CAD build for the part. Positions are in the model's coordinates, mm. Round coordinates to 2 decimals unless told otherwise and drop trailing zeros. Loops run counter-clockwise (first coordinate to the right, second up) from the corner with the lowest first, then second, coordinate; pieces in that order, holes last.
from build123d import *

# Parameters (mm, degrees)
CYLINDER080_R     = 1.5
CYLINDER080_DEPTH = 10
CYLINDER075_R     = 2.579687
CYLINDER075_DEPTH = 56.5
CYLINDER076_R     = 2.579687
CYLINDER076_DEPTH = 55.5
BOX006_W          = 6.35
BOX006_H          = 15
BOX006_DEPTH      = 10
FILLET005_R       = 1
BOX005_W          = 6.35
BOX005_H          = 15
BOX005_DEPTH      = 10
FILLET004_R       = 1
BOX004_W          = 68
BOX004_H          = 15
BOX004_DEPTH      = 1.01
FILLET003_R       = 2


with BuildPart() as shieldcrosshole004:
    # Cylinder080 → Cylinder080 (new body)
    with BuildSketch(Plane(origin=(105, 116, 34), x_dir=(1, 0, 0), z_dir=(0, 0, 1))):
        Circle(CYLINDER080_R)
    extrude(amount=CYLINDER080_DEPTH)


with BuildPart() as threaded027:
    # Cylinder075 → Cylinder075 (new body)
    with BuildSketch(Plane(origin=(73.25, 179.75, 4), x_dir=(1, 0, 0), z_dir=(0, 0, 1))):
        Circle(CYLINDER075_R)
    extrude(amount=CYLINDER075_DEPTH)


with BuildPart() as threaded028:
    # Cylinder076 → Cylinder076 (new body)
    with BuildSketch(Plane(origin=(136.75, 179.75, 4), x_dir=(1, 0, 0), z_dir=(0, 0, 1))):
        Circle(CYLINDER076_R)
    extrude(amount=CYLINDER076_DEPTH)


with BuildPart() as fillet005:
    # Box006 → Box006 (new body)
    with BuildSketch(Plane(origin=(70.075, 175.825, 36), x_dir=(1, 0, 0), z_dir=(0, 0, 1))):
        with Locations((3.175, 7.5)):
            Rectangle(BOX006_W, BOX006_H)
    extrude(amount=BOX006_DEPTH)

    # Fillet005
    fillet005_edges = [fillet005.edges().sort_by_distance(p)[0] for p in [
        (70.075, 175.825, 41),
        (76.425, 175.825, 41),
    ]]
    fillet(fillet005_edges, radius=FILLET005_R)


with BuildPart() as fillet005_1:
    # Fillet005 placement: moved
    add(fillet005.part.moved(Location((63.5, 0, 0))))


with BuildPart() as fusion033:
    # Box005 → Box005 (new body)
    with BuildSketch(Plane(origin=(70.075, 175.825, 36), x_dir=(1, 0, 0), z_dir=(0, 0, 1))):
        with Locations((3.175, 7.5)):
            Rectangle(BOX005_W, BOX005_H)
    extrude(amount=BOX005_DEPTH)

    # Fillet004
    fillet004_edges = [fusion033.edges().sort_by_distance(p)[0] for p in [
        (70.075, 175.825, 41),
        (76.425, 175.825, 41),
    ]]
    fillet(fillet004_edges, radius=FILLET004_R)

    # Fusion033: union Threaded027, Threaded028, Fillet005
    add(threaded027.part)
    add(threaded028.part)
    add(fillet005_1.part)


with BuildPart() as shieldbar003:
    # Box004 → Box004 (new body)
    with BuildSketch(Plane(origin=(71, 169.75, 39), x_dir=(1, 0, 0), z_dir=(0, 0, 1))):
        with Locations((34, 7.5)):
            Rectangle(BOX004_W, BOX004_H)
    extrude(amount=BOX004_DEPTH)

    # Fillet003
    fillet003_edges = [shieldbar003.edges().sort_by_distance(p)[0] for p in [
        (71, 169.75, 39.505),
        (71, 184.75, 39.505),
        (139, 169.75, 39.505),
        (139, 184.75, 39.505),
    ]]
    fillet(fillet003_edges, radius=FILLET003_R)

    # Cut004: cut Fusion033
    add(fusion033.part, mode=Mode.SUBTRACT)


with BuildPart() as shieldbar003_1:
    # Cut004 placement: moved
    add(shieldbar003.part.moved(Location((0, -63.5, 0))))

    # Cut006: cut ShieldCrossHole004
    add(shieldcrosshole004.part, mode=Mode.SUBTRACT)


solid = shieldbar003_1.part
Item 1: Cut at B-B (z = 39.8). List the corners of the cut face in (x, y) (3 decimals).
Verdict:
outline: (71, 108.25) arc R2 ccw to (73, 106.25) - (137, 106.25) arc R2 ccw to (139, 108.25) - (139, 112.328) arc R1 cw to (138.925, 112.325) - (134.575, 112.325) arc R1 cw to (133.575, 113.325) - (133.575, 121.25) - (76.425, 121.25) - (76.425, 113.325) arc R1 cw to (75.425, 112.325) - (71.075, 112.325) arc R1 cw to (71, 112.328) - close; hole circle Ø3 at (105, 116)
Item 2: Cut at A-A (x = 105). List the corners of the cut face in (y, z), plus the area to 3 significant figures.
Verdict:
outline: (106.25, 39) - (114.5, 39) - (114.5, 40.01) - (106.25, 40.01) - close; (117.5, 39) - (121.25, 39) - (121.25, 40.01) - (117.5, 40.01) - close
area: 12.1 mm2
Item 3: Cut at C-C (y = 116). List the corners of the cut face in (x, z) (3 decimals).
Verdict:
outline: (76.425, 39) - (103.5, 39) - (103.5, 40.01) - (76.425, 40.01) - close; (106.5, 39) - (133.575, 39) - (133.575, 40.01) - (106.5, 40.01) - close
Item 4: Mould opens along X. For faces 1 (the cylindrical face through (138.4, 106.82, 39.51)), 2 (the flat face through (105, 114, 40.01)), 3 (the cylindrical face through (71.57, 106.85, 39.51)), 4 (the cylindrical face through (104.805, 117.487, 39.498)) say: released by +X, released by -X, zero draft, split by the parting line, or undercut.
Verdict:
face 1: released by +X
face 2: zero draft
face 3: released by -X
face 4: undercut
Item 5: Wall check: L1, parallel to Y at x = 105, z = 39.8; L2, parallel to X at y = 116, z = 39.55 (3 decimals); L3, parallel to X at y = 114.25, z = 39.3 (3 decimals). Give the ranges that are in metal, low to high.
Verdict:
L1: y = 106.25 to 114.5, 117.5 to 121.25
L2: x = 76.425 to 103.5, 106.5 to 133.575
L3: x = 76.425 to 133.575
